Design review of the part built by this model. Coordinates are the model's own, in mm. A direction names the side the tool comes from. Coordinates: 2 decimals unless noted, no trailing zeros. Loops run counter-clockwise (first coordinate to the right, second up) from the corner with the lowest first, then second, coordinate; pieces in that order, holes last. Notation, with made-up numbers: (4, 45) -> (57, 45) arc R23 ccw to (57, 72) -> close; hole circle Ø4 at (22.5, -13.5). An arc over 180 degrees is marked (long way). Answer as a JSON object with one key per item and string values.
```python
from build123d import *

# Parameters (mm, degrees)
BOSS_EXTRUDE1_DEPTH = 1.5
SKETCH2_W           = 2
SKETCH2_H           = 1.5
BOSS_EXTRUDE2_DEPTH = 0.01


with BuildPart() as part:
    # Sketch1 → Boss-Extrude1 (new body)
    with BuildSketch(Plane(origin=(0, 0, 0), x_dir=(1, 0, 0), z_dir=(0, 1, 0))):
        with BuildLine():
            Line((-7.5, -20.227321531), (-7.5, 19.772678469))
            Line((-7.5, 19.772678469), (-3.4, 19.772678469))
            ThreePointArc((-3.4, 19.772678469), (-3.046446609, 19.919125079), (-2.9, 20.272678469))
            Line((-2.9, 20.272678469), (-2.9, 20.772678469))
            Line((-2.9, 20.772678469), (-0.9, 20.772678469))
            Line((-0.9, 20.772678469), (-0.9, 20.272678469))
            ThreePointArc((-0.9, 20.272678469), (-0.753553391, 19.919125079), (-0.4, 19.772678469))
            Line((-0.4, 19.772678469), (0.4, 19.772678469))
            ThreePointArc((0.4, 19.772678469), (0.753553391, 19.919125079), (0.9, 20.272678469))
            Line((0.9, 20.272678469), (0.9, 20.772678469))
            Line((0.9, 20.772678469), (2.9, 20.772678469))
            Line((2.9, 20.772678469), (2.9, 20.272678469))
            ThreePointArc((2.9, 20.272678469), (3.046446609, 19.919125079), (3.4, 19.772678469))
            Line((3.4, 19.772678469), (7.5, 19.772678469))
            Line((7.5, 19.772678469), (7.5, -20.227321531))
            Line((7.5, -20.227321531), (3.4, -20.227321531))
            ThreePointArc((3.4, -20.227321531), (3.046446609, -20.37376814), (2.9, -20.727321531))
            Line((2.9, -20.727321531), (2.9, -21.227321531))
            Line((2.9, -21.227321531), (0.9, -21.227321531))
            Line((0.9, -21.227321531), (0.9, -20.727321531))
            ThreePointArc((0.9, -20.727321531), (0.753553391, -20.37376814), (0.4, -20.227321531))
            Line((0.4, -20.227321531), (-0.4, -20.227321531))
            ThreePointArc((-0.4, -20.227321531), (-0.753553391, -20.37376814), (-0.9, -20.727321531))
            Line((-0.9, -20.727321531), (-0.9, -21.227321531))
            Line((-0.9, -21.227321531), (-2.9, -21.227321531))
            Line((-2.9, -21.227321531), (-2.9, -20.727321531))
            ThreePointArc((-2.9, -20.727321531), (-3.046446609, -20.37376814), (-3.4, -20.227321531))
            Line((-3.4, -20.227321531), (-7.5, -20.227321531))
        make_face()
    extrude(amount=BOSS_EXTRUDE1_DEPTH)

    # Sketch2 → Boss-Extrude2 (add)
    with BuildSketch(Plane.XZ):
        with Locations((-1.95, -17.177321531)):
            Rectangle(SKETCH2_W, SKETCH2_H)
        with Locations((1.95, -17.177321531)):
            Rectangle(SKETCH2_W, SKETCH2_H)
        with Locations((-1.95, -14.177321531)):
            Rectangle(SKETCH2_W, SKETCH2_H)
        with Locations((1.95, -14.177321531)):
            Rectangle(SKETCH2_W, SKETCH2_H)
        with Locations((-1.95, -11.177321531)):
            Rectangle(SKETCH2_W, SKETCH2_H)
        with Locations((-1.95, -8.177321531)):
            Rectangle(SKETCH2_W, SKETCH2_H)
        with Locations((-1.95, -5.177321531)):
            Rectangle(SKETCH2_W, SKETCH2_H)
        with Locations((-1.95, -2.177321531)):
            Rectangle(SKETCH2_W, SKETCH2_H)
        with Locations((-1.95, 0.822678469)):
            Rectangle(SKETCH2_W, SKETCH2_H)
        with Locations((-1.95, 3.822678469)):
            Rectangle(SKETCH2_W, SKETCH2_H)
        with Locations((-1.95, 6.822678469)):
            Rectangle(SKETCH2_W, SKETCH2_H)
        with Locations((1.95, 6.822678469)):
            Rectangle(SKETCH2_W, SKETCH2_H)
        with Locations((-1.95, 9.822678469)):
            Rectangle(SKETCH2_W, SKETCH2_H)
        with Locations((1.95, 9.822678469)):
            Rectangle(SKETCH2_W, SKETCH2_H)
    extrude(amount=BOSS_EXTRUDE2_DEPTH)


solid = part.part
```
1) Clearance check with flat-ended pins moving along their axes: pin 1 Ø0.9 at (x, y) = (0, 0.5) entering from -Z; pin 2 Ø0.6 at (y, z) = (0.5, -20.5) entering from -X. State where each tip first meets the part, or that it passes through.
Completed:
{"pin 1": "z = -19.78", "pin 2": "x = -2.91"}
2) Add section B-B, the plane x = -4.5. Give the boundary of the cut face in (y, z), and give its area (3 significant figures).
Completed:
{"outline": "(0, -19.77) -> (1.5, -19.77) -> (1.5, 20.23) -> (0, 20.23) -> close", "area": "60.0 mm²"}
3) For faces 1 (the flat face through (-5, 1, -19.773)), 2 (the flat face through (5, 1, -19.773)), 3 (the flat face through (-2, -0.01, 1)), 4 (the flat face through (-5, 1, 20.227)), list the 3-axis set-ups (+Z, -Z, +X, -X, +Y, -Y) from which the entire face can be reached by the end or side of a thin tool; tool diameter is ignored.
Completed:
{"face 1": "-Z, -X, +Y, -Y", "face 2": "-Z, +X, +Y, -Y", "face 3": "+Z, -Z, +X, -X, -Y", "face 4": "+Z, -X, +Y, -Y"}
4) Add section A-A, the plane y = 0.35. Give the boundary of the cut face in (x, z).
Completed:
{"outline": "(-7.5, -19.77) -> (-3.4, -19.77) arc R0.5 cw to (-2.9, -20.27) -> (-2.9, -20.77) -> (-0.9, -20.77) -> (-0.9, -20.27) arc R0.5 cw to (-0.4, -19.77) -> (0.4, -19.77) arc R0.5 cw to (0.9, -20.27) -> (0.9, -20.77) -> (2.9, -20.77) -> (2.9, -20.27) arc R0.5 cw to (3.4, -19.77) -> (7.5, -19.77) -> (7.5, 20.23) -> (3.4, 20.23) arc R0.5 cw to (2.9, 20.73) -> (2.9, 21.23) -> (0.9, 21.23) -> (0.9, 20.73) arc R0.5 cw to (0.4, 20.23) -> (-0.4, 20.23) arc R0.5 cw to (-0.9, 20.73) -> (-0.9, 21.23) -> (-2.9, 21.23) -> (-2.9, 20.73) arc R0.5 cw to (-3.4, 20.23) -> (-7.5, 20.23) -> close"}
5) Wall thickness on probe 1 along Y at (x, z) = (4, -4); probe 2 along Z at (x, y) = (4.25, 0.85): over which ranges is each line inside the solid? List them lowest first.
Completed:
{"probe 1": "0 to 1.5", "probe 2": "-19.77 to 20.23"}
